Work out the finished part from the listing and answer in its coordinate system (mm). Face numbers are marked on the shaded views. Give positions to 0.01 mm unless a question says otherwise; leave off trailing zeros. Loops run counter-clockwise (first coordinate to the right, second up) from the corner with the lowest first, then second, coordinate; pieces in that order, holes last. Notation, with made-up numbers: (15, 13.5) - (61, 13.5) arc R22 ccw to (61, 35.5) - close; hole circle Ø9 at (41, -3). An arc over 180 degrees is marked (long way). One line per question, with ' | ' between items.
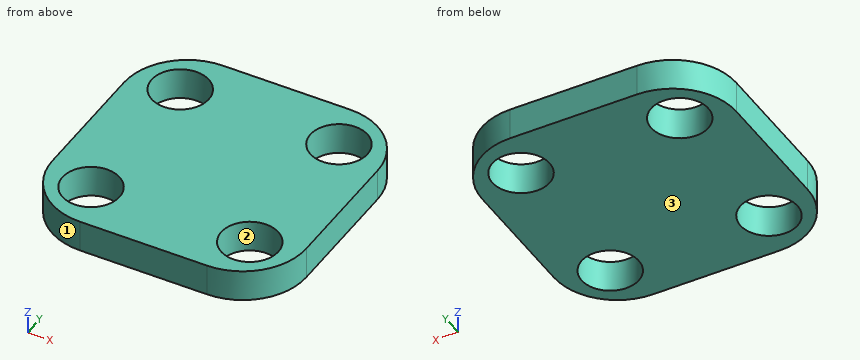
from build123d import *

# Parameters (mm, degrees)
CYLINDER059_R       = 1.8
CYLINDER059_DEPTH   = 20
ARRAY001007_X_COUNT = 2
ARRAY001007_X_PITCH = 10
ARRAY001007_Y_COUNT = 2
ARRAY001007_Y_PITCH = 10
BOX008_W            = 16
BOX008_H            = 16
BOX008_DEPTH        = 2
FILLET014_R         = 4


with BuildPart() as rod_holder_hole_array001:
    # Cylinder059 → Cylinder059 (new body)
    with BuildSketch(Plane(origin=(3, 3, -6), x_dir=(1, 0, 0), z_dir=(0, 0, 1))):
        Circle(CYLINDER059_R)
    extrude(amount=CYLINDER059_DEPTH)

    # Array001007 X: rod holder hole array001 ×2


with BuildPart() as rod_holder_hole_array001_1:
    add(rod_holder_hole_array001.part)
    with Locations(*[(i * ARRAY001007_X_PITCH, 0, 0) for i in range(1, ARRAY001007_X_COUNT)]):
        add(rod_holder_hole_array001.part)

    # Array001007 Y: rod holder hole array001 ×2


with BuildPart() as rod_holder_hole_array001_2:
    add(rod_holder_hole_array001_1.part)
    with Locations(*[(0, i * ARRAY001007_Y_PITCH, 0) for i in range(1, ARRAY001007_Y_COUNT)]):
        add(rod_holder_hole_array001_1.part)


with BuildPart() as rod_cover_fillet:
    # Box008 → Box008 (new body)
    with BuildSketch(Plane.XY):
        with Locations((8, 8)):
            Rectangle(BOX008_W, BOX008_H)
    extrude(amount=BOX008_DEPTH)

    # Cut023005: cut rod holder hole array001
    add(rod_holder_hole_array001_2.part, mode=Mode.SUBTRACT)

    # Fillet014
    fillet014_edges = [rod_cover_fillet.edges().sort_by_distance(p)[0] for p in [
        (0, 0, 1),
        (0, 16, 1),
        (16, 0, 1),
        (16, 16, 1),
    ]]
    fillet(fillet014_edges, radius=FILLET014_R)


solid = rod_cover_fillet.part
1. A flat-ended cylindrical pin translates along its axis: pin 1 (3 mm diameter, centred on x = 3, y = 3, fed in from -Z). Find the tip coordinate at first contact, or state that the pin passes through.
Evaluation:
pin 1: through
2. Consider L1, parallel to X at y = 14.5, z = 1.45; L2, parallel to X at y = 3, z = 1.5. Determine where each line is inside the solid, lowest interval first.
Evaluation:
L1: 0.88 to 2.01, 3.99 to 12.01, 13.99 to 15.12 | L2: 0.13 to 1.2, 4.8 to 11.2, 14.8 to 15.87
3. Find section C-C on y = 1.5. Write down the section's boundary in (x, z), then the cut area to 3 significant figures.
Evaluation:
outline: (0.88, 0) - (2.01, 0) - (2.01, 2) - (0.88, 2) - close; (3.99, 0) - (12.01, 0) - (12.01, 2) - (3.99, 2) - close; (13.99, 0) - (15.12, 0) - (15.12, 2) - (13.99, 2) - close | area: 20.5 mm2
4. Determine the mould class of the marked faces 1, 2 and 3 for opening direction X: +X half, -X half, draft (parallel to the pull), parting line (faces both ways), or undercut.
Evaluation:
face 1: -X half | face 2: undercut | face 3: draft
5. Find section A-A on z = 0.7. Write down the section's boundary in (x, y).
Evaluation:
outline: (0, 4) arc R4 ccw to (4, 0) - (12, 0) arc R4 ccw to (16, 4) - (16, 12) arc R4 ccw to (12, 16) - (4, 16) arc R4 ccw to (0, 12) - close; hole circle Ø3.6 at (3, 3); hole circle Ø3.6 at (3, 13); hole circle Ø3.6 at (13, 3); hole circle Ø3.6 at (13, 13)
6. Find section B-B on x = 3.75. Write down the section's boundary in (y, z), then the cut area to 3 significant figures.
Evaluation:
outline: (0.01, 0) - (1.36, 0) - (1.36, 2) - (0.01, 2) - close; (4.64, 0) - (11.36, 0) - (11.36, 2) - (4.64, 2) - close; (14.64, 0) - (15.99, 0) - (15.99, 2) - (14.64, 2) - close | area: 18.9 mm2
